Work out the finished part from the listing and answer in its coordinate system (mm). A direction names the side the tool comes from. Coordinates: 2 decimals unless noted, no trailing zeros. Order: outer loops, then holes, each group sorted by start corner. A loop starts at its lowest first (then second) coordinate and runs counter-clockwise, first axis right, second up. Notation, with made-up numbers: M -23.75,60 L 23.25,60 A22 cw 23.25,89 Z; hole C 7.25,44.25 d11. An arc over 180 degrees is marked long. Write item = value, one per line. Start each with the question number.
Q1. Straight lines are drawn through the part: line 1 along Y through (x, z) = (0, 13.5); line 2 along Y through (x, z) = (0, 2.3) (3 decimals); line 3 along Z through (x, y) = (-19, 9.5). For each, find the intervals that lie inside material, in ascending order.
Q2. Determine the mould class of faces 1 (the flat face through (0, 5, 25)), 2 (the flat face through (2, -2, 5)), 3 (the cylindrical face through (23.846, 7.509, 10.353)) for opening direction X: released by +X, released by -X, zero draft, split by the parting line, or undercut.
Q3. A tool of negligible diameter and unlimited length cuts with its end or side. For faces 4 (the cylindrical face through (2.5, 0.8, 2.5)), 5 (the cylindrical face through (-0.59, 4.46, 15.14)), from which of +Z, -Z, +X, -X, +Y, -Y can it reach the whole face along a straight path? Write none if from no direction.
Q4. Each of these flat-tipped pins is pushed along its axis until it touches: P1, Ø10, axis at x = 2, z = 5, coming from the -Y side; P2, Ø12, axis at y = 3, z = 4, coming from the +X side; P3, Ø2, axis at y = 8, z = 8.5, coming from the +X side; P4, Ø5, axis at y = 12, z = 11.5, coming from the +X side. Where does it stop, or does it pass through?
Q5. Find section A-A on y = 0. Give the vertices of the cut face in (x, z) (3 decimals), and give its area (3 significant figures).
Q6. Find section C-C on z = 13.5. Give the vertices of the cut face in (x, y), and give its area (3 significant figures).
```python
from build123d import *

# Parameters (mm, degrees)
F0_R     = 25
F1_DEPTH = 25
F2_R     = 2.625
F3_DEPTH = 25
F4_R     = 4.5
F5_DEPTH = 20
F6_R     = 4


with BuildPart() as f1:
    # F0 (on Top) → F1 (new body)
    with BuildSketch(Plane.XY):
        Circle(F0_R)
    extrude(amount=F1_DEPTH)

    # F2 (on face) → F3 (cut)
    with BuildSketch(Plane.XY.offset(25)):
        Circle(F2_R)
    extrude(amount=-F3_DEPTH, mode=Mode.SUBTRACT)

    # F4 (on face) → F5 (cut)
    with BuildSketch(Plane.XY.offset(25)):
        Circle(F4_R)
    extrude(amount=-F5_DEPTH, mode=Mode.SUBTRACT)

    # F6
    f6_edges = [f1.edges().sort_by_distance(p)[0] for p in [
        (-25, 0, 25),
    ]]
    fillet(f6_edges, radius=F6_R)


solid = f1.part
```
Findings below:
q1.line_1 = -25 to -4.5, 4.5 to 25
q1.line_2 = -25 to -2.625, 2.625 to 25
q1.line_3 = 0 to 24.99
q2.face_1 = zero draft
q2.face_2 = undercut
q2.face_3 = split by the parting line
q3.face_4 = +Z, -Z
q3.face_5 = +Z
q4.P1 = -25
q4.P2 = 25
q4.P3 = 24
q4.P4 = 23.12
q5.outline = M -25,0 L -2.625,0 L -2.625,5 L -4.5,5 L -4.5,25 L -21,25 A4 ccw -25,21 Z; M 2.625,0 L 25,0 L 25,21 A4 ccw 21,25 L 4.5,25 L 4.5,5 L 2.625,5 Z
q5.area = 1,040 mm^2
q6.outline = C 0,0 d50; hole C 0,0 d9
q6.area = 1,900 mm^2
